```python
from build123d import *

# Parameters (mm, degrees)
F0_W      = 50
F0_H      = 50
F1_DEPTH  = 50
F2_R      = 5
F3_R      = 5
F4_DEPTH  = 1
F5_R      = 5
F6_DEPTH  = 1
F7_R      = 5
F8_DEPTH  = 1
F9_R      = 5
F10_DEPTH = 1
F11_R     = 5
F12_DEPTH = 1
F13_R     = 5
F14_DEPTH = 1


with BuildPart() as f1:
    # F0 (on Front) → F1 (new body)
    with BuildSketch(Plane.XZ):
        with Locations((25, 25)):
            Rectangle(F0_W, F0_H)
    extrude(amount=F1_DEPTH)

    # F2
    f2_edges = [f1.edges().sort_by_distance(p)[0] for p in [
        (50, -50, 25),
        (50, -25, 50),
        (25, -50, 50),
        (25, -50, 0),
        (50, -25, 0),
        (50, 0, 25),
        (25, 0, 50),
        (0, -25, 50),
        (0, 0, 25),
        (25, 0, 0),
        (0, -25, 0),
        (0, -50, 25),
    ]]
    fillet(f2_edges, radius=F2_R)

    # F3 (on face) → F4 (cut)
    with BuildSketch(Plane.XZ.offset(50)):
        with Locations((25, 25)):
            Circle(F3_R)
    extrude(amount=-F4_DEPTH, mode=Mode.SUBTRACT)

    # F5 (on face) → F6 (cut)
    with BuildSketch(Plane(origin=(0, 0, 0), x_dir=(-1, 0, 0), z_dir=(0, 1, 0))):
        with Locations((-37, 37)):
            Circle(F5_R)
        with Locations((-13, 37)):
            Circle(F5_R)
        with Locations((-37, 25)):
            Circle(F5_R)
        with Locations((-13, 25)):
            Circle(F5_R)
        with Locations((-13, 13)):
            Circle(F5_R)
        with Locations((-37, 13)):
            Circle(F5_R)
    extrude(amount=-F6_DEPTH, mode=Mode.SUBTRACT)

    # F7 (on face) → F8 (cut)
    with BuildSketch(Plane.XY.offset(50)):
        with Locations((37, -13)):
            Circle(F7_R)
        with Locations((37, -37)):
            Circle(F7_R)
        with Locations((25, -25)):
            Circle(F7_R)
        with Locations((13, -13)):
            Circle(F7_R)
        with Locations((13, -37)):
            Circle(F7_R)
    extrude(amount=-F8_DEPTH, mode=Mode.SUBTRACT)

    # F9 (on face) → F10 (cut)
    with BuildSketch(Plane(origin=(0, 0, 0), x_dir=(1, 0, 0), z_dir=(0, 0, -1))):
        with Locations((37, 37)):
            Circle(F9_R)
        with Locations((13, 13)):
            Circle(F9_R)
    extrude(amount=-F10_DEPTH, mode=Mode.SUBTRACT)

    # F11 (on face) → F12 (cut)
    with BuildSketch(Plane.YZ.offset(50)):
        with Locations((-37, 37)):
            Circle(F11_R)
        with Locations((-25, 25)):
            Circle(F11_R)
        with Locations((-13, 13)):
            Circle(F11_R)
    extrude(amount=-F12_DEPTH, mode=Mode.SUBTRACT)

    # F13 (on face) → F14 (cut)
    with BuildSketch(Plane(origin=(0, 0, 0), x_dir=(0, -1, 0), z_dir=(-1, 0, 0))):
        with Locations((37, 37)):
            Circle(F13_R)
        with Locations((37, 13)):
            Circle(F13_R)
        with Locations((13, 13)):
            Circle(F13_R)
        with Locations((13, 37)):
            Circle(F13_R)
    extrude(amount=-F14_DEPTH, mode=Mode.SUBTRACT)


solid = f1.part
```
Geometry check sheet. Reference: the model listing, model coordinates, mm. A direction names the side the tool comes from. Round coordinates to 2 decimals unless told otherwise and drop trailing zeros. Order: outer loops, then holes, each group sorted by start corner. A loop starts at its lowest first (then second) coordinate and runs counter-clockwise, first axis right, second up. Notation, with made-up numbers: (59, 42) - (77, 42) arc R10 ccw to (77, 52) - close; hole circle Ø1 at (-27.75, 1.5). An arc over 180 degrees is marked (long way). Use a Markdown table: item, result. Add a question column.
1) Set-up check for faces 5 (the flat face through (37, -37, 1)), 6 (the cylindrical face through (0.493, -15.688, 41.216)), 7 (the cylindrical face through (15.688, -32.784, 49.507)): record each of +Z, -Z, +X, -X, +Y, -Y from which the full face is reachable in a straight line by a thin tool's end or side.
2) Section check D-D (x = 26.5). Record the cut outline in (y, z).
3) Mould release check, pull along Y, two halves, no side actions. Record for faces 1 (the flat face through (13, -1, 25)), 2 (the cylindrical face through (10.693, -0.493, 20.564)), 3 (the flat face through (13, -13, 49)), 4 (the flat face through (25, -49, 25)): released by +Y, released by -Y, zero draft, split by the parting line, or undercut.
4) Section check A-A (z = 13). Record the cut outline in (x, y), then the cut area to 3 significant figures.
5) Gauge pin test, flat ends, axial feed: P1, Ø16, axis at y = -13, z = 13, coming from the +X side; P2, Ø3, axis at x = 36.5, y = -13.5, coming from the +Z side; P3, Ø5, axis at x = 36, y = -36.5, coming from the -Z side; P4, Ø5, axis at x = 23.5, z = 25.5, coming from the -Y side. Record the tip position at first contact, or that the pin passes through.
6) Thickness scan on line 1 along Z through (x, y) = (0.8, -37); line 2 along Z through (x, y) = (0.4, -37); line 3 along Y through (x, z) = (39.5, 41). Record the ranges inside material, lowest first.
Established:
| question | item | result |
|---|---|---|
| 1 | face 5 | -Z |
| 1 | face 6 | -X |
| 1 | face 7 | +Z |
| 2 | outline | (-50, 5) arc R5 ccw to (-45, 0) - (-5, 0) arc R5 ccw to (0, 5) - (0, 45) arc R5 ccw to (-5, 50) - (-20.23, 50) - (-20.23, 49) - (-29.77, 49) - (-29.77, 50) - (-45, 50) arc R5 ccw to (-50, 45) - (-50, 29.77) - (-49, 29.77) - (-49, 20.23) - (-50, 20.23) - close |
| 3 | face 1 | released by +Y |
| 3 | face 2 | zero draft |
| 3 | face 3 | undercut |
| 3 | face 4 | released by -Y |
| 4 | outline | (0, -45) arc R5 ccw to (5, -50) - (45, -50) arc R5 ccw to (50, -45) - (50, -18) - (49, -18) - (49, -8) - (50, -8) - (50, -5) arc R5 ccw to (45, 0) - (42, 0) - (42, -1) - (32, -1) - (32, 0) - (18, 0) - (18, -1) - (8, -1) - (8, 0) - (5, 0) arc R5 ccw to (0, -5) - (0, -8) - (1, -8) - (1, -18) - (0, -18) - (0, -32) - (1, -32) - (1, -42) - (0, -42) - close |
| 4 | area | 2,430 mm2 |
| 5 | P1 | x = 50 |
| 5 | P2 | z = 49 |
| 5 | P3 | z = 1 |
| 5 | P4 | y = -49 |
| 6 | line 1 | 2.29 to 8, 18 to 32, 42 to 47.71 |
| 6 | line 2 | 3.04 to 8, 18 to 32, 42 to 46.96 |
| 6 | line 3 | -50 to -1 |
